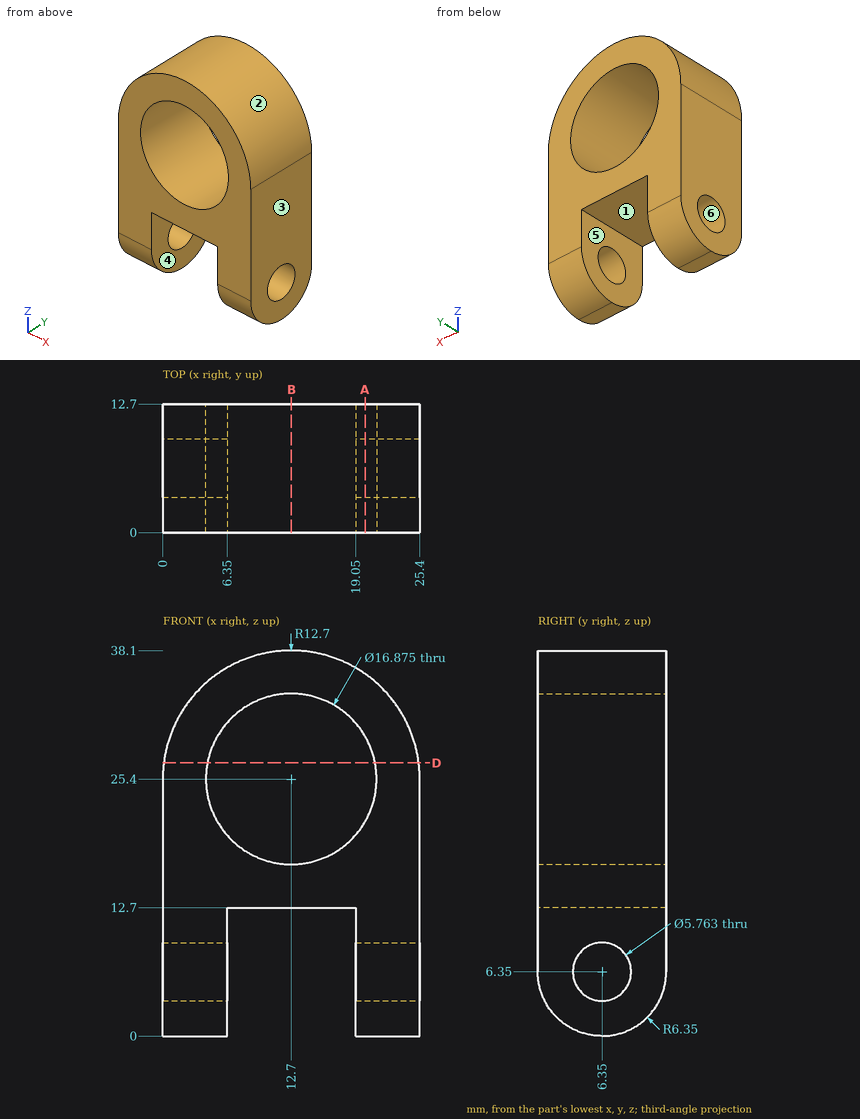
Check sheet for the drawn part. Datum: minimum x, y, z corner. Units: mm. A direction names the side the tool comes from. Give positions to 0.01 mm unless a question says otherwise; leave off trailing zeros. Write each loop counter-clockwise with the first axis right and the second up, starting at its lowest first coordinate (ties: lowest second). Pieces come first, ordered by that corner, then holes.
(1) Mould release check, pull along X, two halves, no side actions. Record for the marked faces 3, 4, 5 and 6: +X half, -X half, draft (parallel to the pull), parting line (faces both ways), or undercut.
(2) Cross-section at D-D (z = 27). Enter the section's corners in (x, y) (1 decimal), plus the area to 3 significant figures.
(3) Gauge pin test, flat end, axial feed: pin 1 (2 mm diameter, centred on x = 22, y = 10.5, fed in from -Z) (1 decimal). Record the tip position at first contact, or that the pin passes through.
(4) Cross-section at A-A (x = 20). State how many separate pieces and enclosed holes the cut face has, plus the area to 3 significant figures.
(5) Material ranges on line 1 (Z direction, x = 12.7, y = 7.5); line 2 (X direction, y = 4, z = 4); line 3 (Z direction, x = 23.25, y = 6.35) (1 decimal), recorded low to high.
(6) Cross-section at B-B (x = 12.7). Enter the section's corners in (y, z).
(7) Access from +Z, -Z, +X, -X, +Y, -Y to the whole of each face (thin tool, end or side, straight path). Record for the marked faces 1 and 2.
Worked out:
1. face 3: +X half
1. face 4: undercut
1. face 5: undercut
1. face 6: draft
2. outline: (0.1, 0) - (4.4, 0) - (4.4, 12.7) - (0.1, 12.7) - close; (21, 0) - (25.3, 0) - (25.3, 12.7) - (21, 12.7) - close
2. area: 110 mm2
3. pin 1: stops at z = 0.8
4. separate pieces: 2
4. enclosed holes: 1
4. area: 304 mm2
5. line 1: z = 12.7 to 16.96, 33.84 to 38.1
5. line 2: x = 0 to 6.35, 19.05 to 25.4
5. line 3: z = 0 to 3.5, 9.2 to 32.5
6. outline: (0, 12.7) - (12.7, 12.7) - (12.7, 16.96) - (0, 16.96) - close; (0, 33.84) - (12.7, 33.84) - (12.7, 38.1) - (0, 38.1) - close
7. face 1: -Z, +Y, -Y
7. face 2: +Z, +Y, -Y
